Answer from the drawing. Dimensions are ordinates in mm from the lowest x, y and z of the part. A direction names the side the tool comes from. Give positions to 0.01 mm unless a question says otherwise; leave off trailing zeros. Write each loop counter-clockwise with the first axis right and the second up, starting at its lowest first coordinate (ties: lowest second). Pieces come first, ordered by that corner, then holes. Notation, with made-up numbers: (-18.5, 72.25) - (-3.5, 72.25) arc R30 ccw to (-3.5, 104.25) - close; hole circle Ø2 at (82.5, 24.5). An arc over 180 degrees is marked (long way). Answer as a JSON object with one key per item and string values. Group by question number.
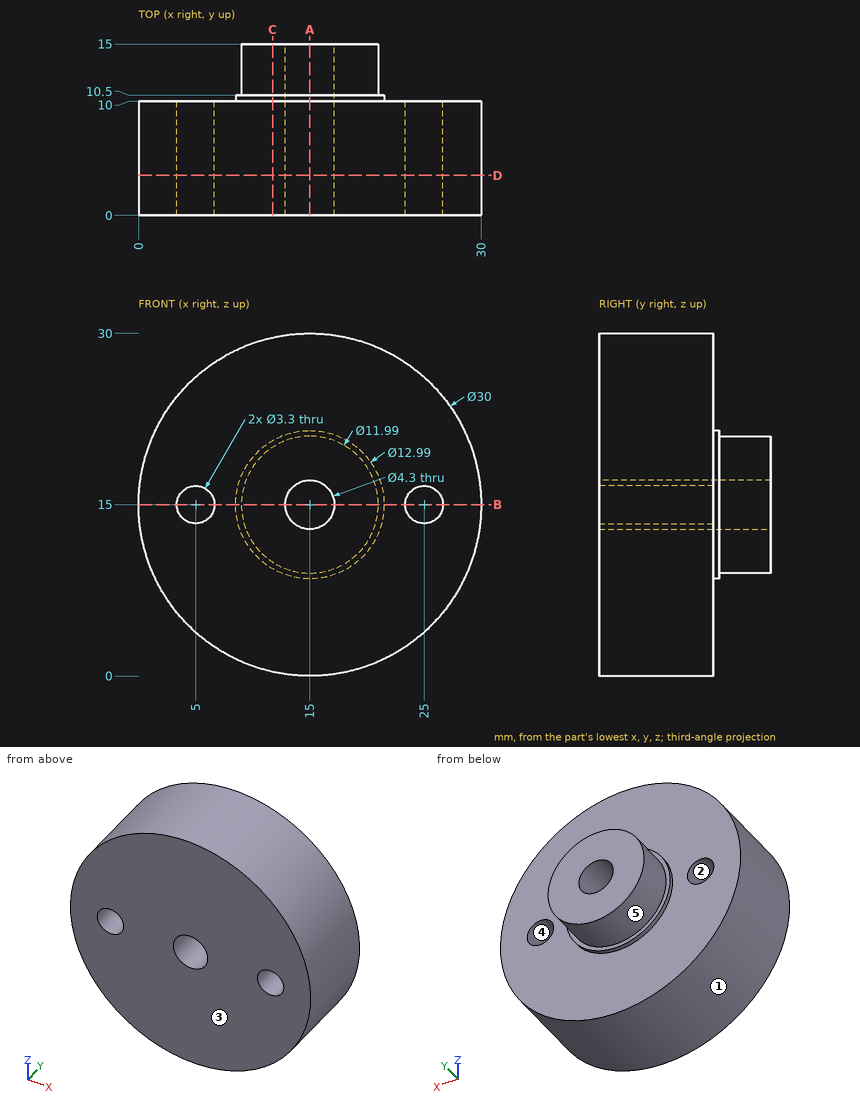
1) Find the intervals of material crossed by line 1 (X direction, y = 7, z = 15); line 2 (X direction, y = 1.25, z = 16.5); line 3 (Y direction, x = 5.75, z = 10), in increasing order. Write a range as [from, to].
2) Find section A-A, the plane x = 15. Write down the section's boundary in (y, z) (3 decimals), and give its area (3 significant figures).
3) For a pull along Z with two mould halves and no side action, classify the marked faces 1, 2 and 3 as released by +Z, released by -Z, zero draft, split by the parting line, or undercut.
4) Find section D-D, the plane y = 3.5. Write down the section's boundary in (x, z), and give its area (3 significant figures).
5) Flat-ended cylindrical pins translate along their axes: pin 1 Ø2 at (y, z) = (10.5, 21.5) entering from -X; pin 2 Ø4 at (y, z) = (9.5, 18.5) entering from +X; pin 3 Ø1.5 at (y, z) = (6.5, 10.5) entering from -X. Find the tip coordinate at first contact, or state that the pin passes through.
6) Which of the six approach directions +Z, -Z, +X, -X, +Y, -Y give full straight-line access (tool end or side, diameter ignored) to the marked faces 4 and 5?
7) Find section C-C, the plane x = 11.75. Write down the section's boundary in (y, z).
8) Find section B-B, the plane z = 15. Write down the section's boundary in (x, y) (3 decimals), and give its area (3 significant figures).
Values follow:
{
 "1": {"line 1": "x = [0, 3.35], [6.65, 12.85], [17.15, 23.35], [26.65, 30]", "line 2": "x = [0.08, 4.31], [5.69, 13.46], [16.54, 24.31], [25.69, 29.92]", "line 3": "y = [0, 10]"},
 "2": {"outline": "(0, 0) - (10, 0) - (10, 8.505) - (10.5, 8.505) - (10.5, 9.005) - (15, 9.005) - (15, 12.85) - (0, 12.85) - close; (0, 17.15) - (15, 17.15) - (15, 20.995) - (10.5, 20.995) - (10.5, 21.495) - (10, 21.495) - (10, 30) - (0, 30) - close", "area": "296 mm2"},
 "3": {"face 1": "split by the parting line", "face 2": "undercut", "face 3": "zero draft"},
 "4": {"outline": "circle Ø30 at (15, 15); hole circle Ø3.3 at (5, 15); hole circle Ø4.3 at (15, 15); hole circle Ø3.3 at (25, 15)", "area": "675 mm2"},
 "5": {"pin 1": "stops at x = 1.1", "pin 2": "stops at x = 29.92", "pin 3": "stops at x = 0.48"},
 "6": {"face 4": "+Y, -Y", "face 5": "+Y"},
 "7": {"outline": "(0, 0.36) - (10, 0.36) - (10, 9.38) - (10.5, 9.38) - (10.5, 9.96) - (15, 9.96) - (15, 20.04) - (10.5, 20.04) - (10.5, 20.62) - (10, 20.62) - (10, 29.64) - (0, 29.64) - close"},
 "8": {"outline": "(0, 0) - (3.35, 0) - (3.35, 10) - (0, 10) - close; (6.65, 0) - (12.85, 0) - (12.85, 15) - (9.005, 15) - (9.005, 10.5) - (8.505, 10.5) - (8.505, 10) - (6.65, 10) - close; (17.15, 0) - (23.35, 0) - (23.35, 10) - (21.495, 10) - (21.495, 10.5) - (20.995, 10.5) - (20.995, 15) - (17.15, 15) - close; (26.65, 0) - (30, 0) - (30, 10) - (26.65, 10) - close", "area": "230 mm2"}
}
